Source: three-view drawing plus pictorial views. Frame: mm from the lowest corner of the part. Give positions to 0.01 mm unless a question says otherwise; leave off trailing zeros. Loops run counter-clockwise (first coordinate to the right, second up) from the corner with the lowest first, then second, coordinate; pieces in that order, holes last. Notation, with made-up numbers: (40, -21) - (62, -21) arc R20 ccw to (62, -12) - close; hole circle Ø4 at (89, 44.25). An arc over 180 degrees is marked (long way). Answer in a Markdown table with one row per item.
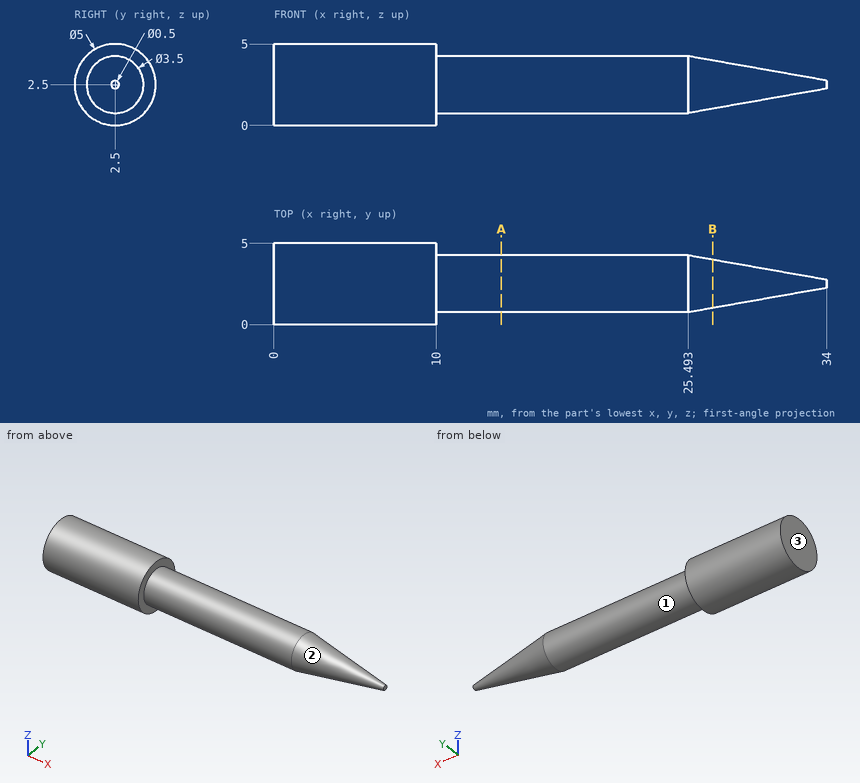
Q1. Cut plane B-B (x = 27). Output: boundary loops of the cut face in (y, z).
Check values:
| item | result |
|---|---|
| outline | circle Ø2.97 at (2.5, 2.5) |
Q2. Material intervals for line 1 along X through (y, z) = (2.25, 0.35); line 2 along Y through (x, z) = (22.5, 2.5); line 3 along Z through (x, y) = (9, 2.35), sorted ascending.
Check values:
| item | result |
|---|---|
| line 1 | 0 to 10 |
| line 2 | 0.75 to 4.25 |
| line 3 | 0 to 5 |
Q3. Cut plane A-A (x = 14). Output: boundary loops of the cut face in (y, z), and give its area (3 significant figures).
Check values:
| item | result |
|---|---|
| outline | circle Ø3.5 at (2.5, 2.5) |
| area | 9.62 mm² |
Q4. Draft query along X for the marked faces 1, 2 and 3. Return one class per face: pulls with the +X half, pulls with the -X half, needs draft (parallel to the pull), parting line crosses it, or undercut.
Check values:
| item | result |
|---|---|
| face 1 | needs draft |
| face 2 | pulls with the +X half |
| face 3 | pulls with the -X half |
